Design review of the part built by this model. Coordinates are the model's own, in mm. Give positions to 0.01 mm unless a question says otherwise; leave off trailing zeros. Write each loop counter-clockwise with the first axis right and the second up, starting at its lowest first coordinate (ties: lowest second). Pieces come first, ordered by that corner, then holes. Notation, with made-up numbers: M 27.25,74.5 L 46.25,74.5 A27 cw 46.25,109.5 Z; hole C 57,-30.75 d7. An arc over 180 degrees is marked long. Use one line per item in the form item = value. Start each with the question number.
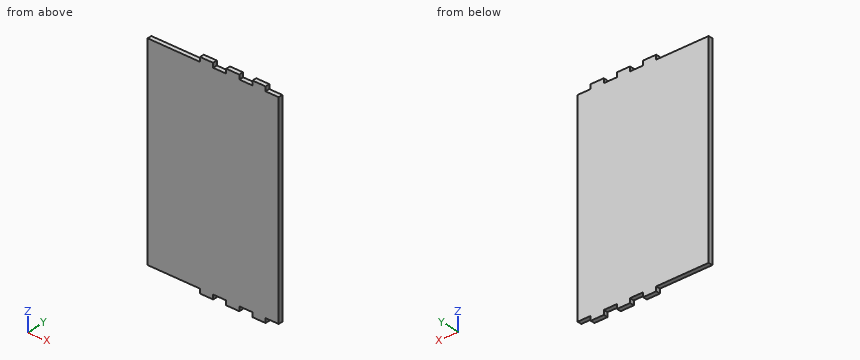
Autodesk Inventor part; units mm, degrees
ref_plane "YZ Plane" through (0, 0, 0) normal (1, 0, 0) x (0, 1, 0)
ref_plane "XZ Plane" through (0, 0, 0) normal (0, 1, 0) x (-1, 0, 0)
ref_plane "XY Plane" through (0, 0, 0) normal (0, 0, 1) x (1, 0, 0)
sketch "Sketch1" plane through (0, 0, 0) normal (0, 1, 0) x (-1, 0, 0)
  line L0 (95.25, 146.05) -> (-95.25, 146.05)
  line L1 (-95.25, 146.05) -> (-95.25, -146.05)
  line L2 (-95.25, -146.05) -> (95.25, -146.05)
  line L3 (95.25, -146.05) -> (95.25, 146.05)
  line L4 (95.25, 146.05) -> (-95.25, -146.05) construction
  line L5 (-95.25, 146.05) -> (95.25, -146.05) construction
  line L6 (95.25, -146.05) -> (76.2, -146.05)
  line L7 (76.2, -146.05) -> (76.2, -152.4)
  line L8 (76.2, -152.4) -> (95.25, -152.4)
  line L9 (95.25, -152.4) -> (95.25, -146.05)
  line L10 (38.1, -146.05) -> (38.1, -152.4)
  line L11 (57.15, -146.05) -> (38.1, -146.05)
  line L12 (38.1, -152.4) -> (57.15, -152.4)
  line L13 (57.15, -152.4) -> (57.15, -146.05)
  line L14 (0, -146.05) -> (0, -152.4)
  line L15 (19.05, -146.05) -> (0, -146.05)
  line L16 (0, -152.4) -> (19.05, -152.4)
  line L17 (19.05, -152.4) -> (19.05, -146.05)
  line L18 (-38.1, -146.05) -> (-38.1, -152.4)
  line L19 (-19.05, -146.05) -> (-38.1, -146.05)
  line L20 (-38.1, -152.4) -> (-19.05, -152.4)
  line L21 (-19.05, -152.4) -> (-19.05, -146.05)
  line L22 (-76.2, -146.05) -> (-76.2, -152.4)
  line L23 (-57.15, -146.05) -> (-76.2, -146.05)
  line L24 (-76.2, -152.4) -> (-57.15, -152.4)
  line L25 (-57.15, -152.4) -> (-57.15, -146.05)
  line L26 (95.25, 0) -> (-95.25, 0) construction
  line L27 (95.25, 146.05) -> (76.2, 146.05)
  line L28 (76.2, 146.05) -> (76.2, 152.4)
  line L29 (76.2, 152.4) -> (95.25, 152.4)
  line L30 (95.25, 152.4) -> (95.25, 146.05)
  line L31 (57.15, 146.05) -> (38.1, 146.05)
  line L32 (38.1, 146.05) -> (38.1, 152.4)
  line L33 (38.1, 152.4) -> (57.15, 152.4)
  line L34 (57.15, 152.4) -> (57.15, 146.05)
  line L35 (19.05, 146.05) -> (0, 146.05)
  line L36 (0, 146.05) -> (0, 152.4)
  line L37 (0, 152.4) -> (19.05, 152.4)
  line L38 (19.05, 152.4) -> (19.05, 146.05)
  line L39 (-19.05, 146.05) -> (-38.1, 146.05)
  line L40 (-38.1, 146.05) -> (-38.1, 152.4)
  line L41 (-38.1, 152.4) -> (-19.05, 152.4)
  line L42 (-19.05, 152.4) -> (-19.05, 146.05)
  line L43 (-57.15, 146.05) -> (-76.2, 146.05)
  line L44 (-76.2, 146.05) -> (-76.2, 152.4)
  line L45 (-76.2, 152.4) -> (-57.15, 152.4)
  line L46 (-57.15, 152.4) -> (-57.15, 146.05)
  point P0 (0, 0)
  dimension "d0" = 292.1
  dimension "d1" = 190.5
  dimension "d2" = 19.05
  dimension "d3" = 6.35
  dimension "d6" = 38.1
  dimension "d11" = 19.05
  dimension "d12" = 6.35
  dimension "d15" = 38.1
extrude "Extrusion2" add sketch "Sketch1" along normal blind 6.35 contours L3 L2 L1 L0 | L0 L36 L37 L38 | L17 L16 L14 L2 | L0 L40 L41 L42 | L21 L20 L18 L2 | L0 L44 L45 L46 | L25 L24 L22 L2
properties part number "ramp2"
1. We need section A-A (y = 5.25). State the section outline as (x, z) points, and give its area (3 significant figures).
2. We need section B-B (x = 52). State the section outline as (y, z) points, and give its area (3 significant figures).
3. Clearance check with flat-ended pins moving along their axes: pin 1 Ø3 at (y, z) = (3.5, 150.5) entering from -X; pin 2 Ø1.9 at (y, z) = (3, -151) entering from +X; pin 3 Ø3 at (y, z) = (2, 147.5) entering from +X; pin 4 Ø1.9 at (x, y) = (51.5, 2) entering from -Z. State where each tip first meets the part, or that it passes through.
4. To check wall thickness, follow L1, parallel to Z at x = -23.5, y = 4.75. State the ranges of the line that lie inside material, in increasing order.
Answer block:
q1.outline = M -95.25,-146.05 L -19.05,-146.05 L -19.05,-152.4 L 0,-152.4 L 0,-146.05 L 19.05,-146.05 L 19.05,-152.4 L 38.1,-152.4 L 38.1,-146.05 L 57.15,-146.05 L 57.15,-152.4 L 76.2,-152.4 L 76.2,-146.05 L 95.25,-146.05 L 95.25,146.05 L 76.2,146.05 L 76.2,152.4 L 57.15,152.4 L 57.15,146.05 L 38.1,146.05 L 38.1,152.4 L 19.05,152.4 L 19.05,146.05 L 0,146.05 L 0,152.4 L -19.05,152.4 L -19.05,146.05 L -95.25,146.05 Z
q1.area = 56,400 mm^2
q2.outline = M 0,-146.05 L 6.35,-146.05 L 6.35,146.05 L 0,146.05 Z
q2.area = 1,850 mm^2
q3.pin_1 = -19.05
q3.pin_2 = 76.2
q3.pin_3 = 95.25
q3.pin_4 = -146.05
q4.L1 = -146.05 to 146.05
